from build123d import *

# Parameters (mm, degrees)
SKETCH1_W                    = 17.8
SKETCH1_H                    = 19.6
BOSS_EXTRUDE1_DEPTH          = 1.66
FILLET1_R                    = 2.7
F_2_5_2_5_DIAMETER_HOLE1_D   = 2.5
F_1_0_1_DIAMETER_HOLE1_D     = 1
F_1_0_1_DIAMETER_HOLE1_DEPTH = 32
F_1_0_1_DIAMETER_HOLE1_TIP   = 0.30043031
LPATTERN1_COUNT              = 7
LPATTERN1_PITCH              = 2.54
SKETCH9_W                    = 3
SKETCH9_H                    = 3
BOSS_EXTRUDE2_DEPTH          = 1.2
SKETCH10_W                   = 2.5
SKETCH10_H                   = 1.25
SKETCH10_W_2                 = 1.25
SKETCH10_H_2                 = 2.5
BOSS_EXTRUDE3_DEPTH          = 1.2
SKETCH11_W                   = 2.4
SKETCH11_H                   = 1.3
BOSS_EXTRUDE4_DEPTH          = 0.5


with BuildPart() as part:
    # Sketch1 → Boss-Extrude1 (new body)
    with BuildSketch(Plane.XY):
        Rectangle(SKETCH1_W, SKETCH1_H)
    extrude(amount=BOSS_EXTRUDE1_DEPTH)

    # Fillet1
    fillet1_edges = [part.edges().sort_by_distance(p)[0] for p in [
        (-8.9, 9.8, 0.83),
        (8.9, 9.8, 0.83),
        (8.9, -9.8, 0.83),
        (-8.9, -9.8, 0.83),
    ]]
    fillet(fillet1_edges, radius=FILLET1_R)

    # Ø2.5 (2.5) Diameter Hole1 (through all)
    with Locations(Plane.XY.offset(1.66)):
        with Locations((-6.35, 7.1), (6.35, 7.1)):
            Hole(F_2_5_2_5_DIAMETER_HOLE1_D / 2)

    # Ø1.0 (1) Diameter Hole1
    with Locations(Plane(origin=(0, 0, 0), x_dir=(-1, 0, 0), z_dir=(0, 0, -1))):
        with Locations((-1.75, 6.3), (1.75, 6.3)):
            Hole(F_1_0_1_DIAMETER_HOLE1_D / 2, depth=F_1_0_1_DIAMETER_HOLE1_DEPTH)
            with Locations((0, 0, -(F_1_0_1_DIAMETER_HOLE1_DEPTH + F_1_0_1_DIAMETER_HOLE1_TIP / 2))):  # 118° drill point
                Cone(0, F_1_0_1_DIAMETER_HOLE1_D / 2, F_1_0_1_DIAMETER_HOLE1_TIP, mode=Mode.SUBTRACT)

    # Sketch7 → Ø1.0 (1) Diameter Hole2 (revolve, cut)
    with BuildSketch(Plane(origin=(7.62, -7.3, 0), x_dir=(0, 1, 0), z_dir=(1, 0, 0))):
        Polygon((0, 0), (0, 1.96043031), (0.5, 1.66), (0.5, 0), align=None)
    f_1_0_1_diameter_hole2 = revolve(axis=Axis((7.62, -7.3, -6.35), (0, 0, 1)), mode=Mode.SUBTRACT)

    # LPattern1: Ø1.0 (1) Diameter Hole2 ×7
    with Locations(*[(-i * LPATTERN1_PITCH, 0, 0) for i in range(1, LPATTERN1_COUNT)]):
        add(f_1_0_1_diameter_hole2, mode=Mode.SUBTRACT)

    # Sketch9 → Boss-Extrude2 (add)
    with BuildSketch(Plane(origin=(0, 0, 0), x_dir=(-1, 0, 0), z_dir=(0, 0, -1))):
        with Locations((0, -2)):
            Rectangle(SKETCH9_W, SKETCH9_H)
    extrude(amount=BOSS_EXTRUDE2_DEPTH)

    # Sketch10 → Boss-Extrude3 (add)
    with BuildSketch(Plane(origin=(0, 0, 0), x_dir=(-1, 0, 0), z_dir=(0, 0, -1))):
        with Locations((2.7, 1.5)):
            Rectangle(SKETCH10_W, SKETCH10_H)
        with Locations((-6.4, 1.5)):
            Rectangle(SKETCH10_W, SKETCH10_H)
        with Locations((-2.7, 1.5)):
            Rectangle(SKETCH10_W, SKETCH10_H)
        with Locations((6.4, 1.5)):
            Rectangle(SKETCH10_W, SKETCH10_H)
        with Locations((3.8, -1.5)):
            Rectangle(SKETCH10_W_2, SKETCH10_H_2)
        with Locations((6, -1.5)):
            Rectangle(SKETCH10_W_2, SKETCH10_H_2)
    extrude(amount=BOSS_EXTRUDE3_DEPTH)

    # Sketch11 → Boss-Extrude4 (add)
    with BuildSketch(Plane(origin=(0, 0, 0), x_dir=(-1, 0, 0), z_dir=(0, 0, -1))):
        with Locations((4.8, -4.35)):
            Rectangle(SKETCH11_W, SKETCH11_H)
    extrude(amount=BOSS_EXTRUDE4_DEPTH)


solid = part.part
CAD build for the part. Positions are in the model's coordinates, mm. A direction names the side the tool comes from. Give positions to 0.01 mm unless a question says otherwise; leave off trailing zeros. Loops run counter-clockwise (first coordinate to the right, second up) from the corner with the lowest first, then second, coordinate; pieces in that order, holes last. Notation, with made-up numbers: M -19,32 L 34,32 A13 ccw 34,54 Z; hole C 50,-39.75 d1. An arc over 180 degrees is marked long. Answer in a Markdown table with one row per item. Add a question column.
Item 1: Band-saw the part on B-B on z = 1.35. Give the number of separate pieces and of enclosed holes in the cut face, then the cut area to 3 significant figures.
Item 2: Probe probe 1 along Y at (x, z) = (0, 0.95); probe 2 along Y at (x, z) = (6.35, 0.6); probe 3 along Z at (x, y) = (-1, -7). List the from-to ranges inside material, lowest first.
Item 3: Drop flat-ended pins along their axis: P1, Ø1.3, axis at x = -4, z = -0.5, coming from the +Y side; P2, Ø1, axis at x = 6, z = -1, coming from the +Y side (3 decimals); P3, Ø2, axis at x = 6.35, y = 7.1, coming from the -Z side; P4, Ø3, axis at x = 6.5, y = 5, coming from the -Z side. Give the stop position or say it passes through.
Item 4: Band-saw the part on C-C on x = -2.54. Give the cut face in (y, z) (3 decimals).
Item 5: Band-saw the part on D-D on y = 5. Give the cut face in (x, z), then the cut area to 3 significant figures.
Item 6: Tool access for faces 5 (the face through (-1.5, -2, -1)), 6 (the face through (3.95, 1.5, -0.6)), 7 (the face through (6, 2.125, -1)), 8 (the face through (-7.65, 1.5, -0.6)): list every direction of +Z, -Z, +X, -X, +Y, -Y with a clear straight run to the whole face (end or side of a thin tool).
Item 7: Mould opens along Y. For faces 1 (the face through (-2.24, -7.7, 0.82)), 2 (the face through (-3, 2.125, -1)), 3 (the face through (-2.7, 1.5, -1.2)), 4 (the face through (5.1, -7.8, 0.8)) say: +Y half, -Y half, draft (parallel to the pull), parting line (faces both ways), or undercut.
Item 8: Band-saw the part on A-A on x = 0. Give the cut face in (y, z).
Reply:
| question | item | result |
|---|---|---|
| 1 | separate pieces | 1 |
| 1 | enclosed holes | 11 |
| 1 | area | 326 mm^2 |
| 2 | probe 1 | y = -9.8 to -7.8, -6.8 to 9.8 |
| 2 | probe 2 | y = -9.8 to 5.85, 8.35 to 9.8 |
| 2 | probe 3 | z = 0 to 1.66 |
| 3 | P1 | stops at y = 9.8 |
| 3 | P2 | stops at y = 2.125 |
| 3 | P3 | passes through |
| 3 | P4 | stops at z = 0 |
| 4 | outline | M -9.8,0 L -7.8,0 L -7.8,1.66 L -9.8,1.66 Z; M -6.8,0 L 0.875,0 L 0.875,-1.2 L 2.125,-1.2 L 2.125,0 L 9.8,0 L 9.8,1.66 L -6.8,1.66 Z |
| 5 | outline | M -8.9,0 L 8.9,0 L 8.9,1.66 L -8.9,1.66 Z |
| 5 | area | 29.5 mm^2 |
| 6 | face 5 | -Z, -Y |
| 6 | face 6 | -Z, +Y, -Y |
| 6 | face 7 | -Z, +X, -X, +Y |
| 6 | face 8 | -Z, -X, +Y, -Y |
| 7 | face 1 | undercut |
| 7 | face 2 | +Y half |
| 7 | face 3 | draft |
| 7 | face 4 | undercut |
| 8 | outline | M -9.8,0 L -7.8,0 L -7.8,1.66 L -9.8,1.66 Z; M -6.8,0 L -3.5,0 L -3.5,-1.2 L -0.5,-1.2 L -0.5,0 L 9.8,0 L 9.8,1.66 L -6.8,1.66 Z |
